Autodesk Inventor part; units mm, degrees
ref_plane "YZ Plane" through (0, 0, 0) normal (1, 0, 0) x (0, 1, 0)
ref_plane "XZ Plane" through (0, 0, 0) normal (0, 1, 0) x (-1, 0, 0)
ref_plane "XY Plane" through (0, 0, 0) normal (0, 0, 1) x (1, 0, 0)
sketch "Sketch1" plane through (0, 0, 0) normal (0, 0, 1) x (1, 0, 0)
  line L0 (0, 0) -> (3, 0)
  line L1 (3, 0) -> (3, 25)
  line L2 (3, 25) -> (0, 25)
  line L3 (0, 25) -> (0, 0)
  line L4 (34, 25) -> (39, 25)
  line L5 (39, 25) -> (39, 0)
  line L6 (39, 0) -> (34, 0)
  line L7 (34, 0) -> (34, 25)
  line L8 (0, 25) -> (39, 25)
  line L9 (39, 25) -> (39, 42)
  line L10 (39, 42) -> (0, 42)
  line L11 (0, 42) -> (0, 25)
  line L12 (34, 25) -> (36, 25)
  line L13 (36, 25) -> (36, 10)
  line L14 (36, 10) -> (34, 10)
  line L15 (34, 10) -> (34, 25)
  point P0 (3, 25)
  point P1 (34, 25)
  dimension "d0" = 3
  dimension "d1" = 25
  dimension "d2" = 5
  dimension "d3" = 25
  dimension "d4" = 31
  dimension "d5" = 39
  dimension "d6" = 17
  dimension "d70" = 2
  dimension "d71" = 15
extrude "Extrusion1" add sketch "Sketch1" along normal blind 17 contours L3 L2 L1 L0 | L11 L10 L9 L4 L8 L2 | L4 L5 L6 L7 L14 L13
sketch "Sketch2" plane through (39, 0, 0) normal (1, 0, 0) x (0, 0, -1)
  line L0 (-17, 28) -> (-17, 42)
  line L1 (0, 42) -> (-17, 42)
  line L2 (-17, 42) -> (0, 42)
  line L3 (0, 42) -> (-17, 28)
  point P0 (0, 0)
  dimension "d9" = 14
extrude "Extrusion2" cut sketch "Sketch2" against normal up to surface (39 mm away)
sketch "Sketch4" plane through (0, 0, 17) normal (0, 0, 1) x (1, 0, 0)
  line L0 (39, 0) -> (39, 42)
  line L1 (20, 42) -> (0, 42)
  line L2 (0, 42) -> (0, 25)
  line L3 (0, 25) -> (20, 25)
  line L4 (20, 25) -> (20, 42)
  circle A0 centre (15, 33.5) radius 3.5
  circle A1 centre (5, 33.5) radius 3.5
  line L5 (3, 25) -> (34, 25)
  line L6 (3, 25) -> (1, 25)
  point P0 (0, 0)
  dimension "d17" = 17
  dimension "d18" = 7
  dimension "d19" = 7
  dimension "d20" = 8.5
  dimension "d22" = 8.5
  dimension "d23" = 5
  dimension "d48" = 5
  dimension "d49" = 20
extrude "Extrusion4" cut sketch "Sketch4" against normal blind 14 contours A0 | A1
sketch "Sketch5" plane through (0, 0, 3) normal (0, 0, 1) x (1, 0, 0)
  arc A0 (15, 37) -> (15, 37) centre (15, 33.5) ccw
  circle A1 centre (15, 33.5) radius 1.5
  circle A2 centre (5, 33.5) radius 3.5
  circle A3 centre (5, 33.5) radius 1.5
  point P0 (0, 0)
  point P1 (32.4191, 39.5294)
  point P2 (27.5809, 39.5294)
  point P3 (22.4191, 39.5294)
  point P4 (17.5809, 39.5294)
  dimension "d26" = 3
  dimension "d27" = 3
extrude "Extrusion5" cut sketch "Sketch5" against normal up to surface (3 mm away) contours A1 | A3
sketch "Sketch10" plane through (0, 0, 17) normal (0, 0, 1) x (1, 0, 0)
  line L0 (39, 42) -> (0, 42)
  line L1 (39, 42) -> (21, 42)
  line L2 (21, 42) -> (21, 35)
  line L3 (39, 28) -> (0, 28)
  line L4 (21, 35) -> (39, 28)
  line L5 (39, 42) -> (39, 28)
  line L6 (39, 28) -> (39, 42)
  point P0 (0, 0)
  dimension "d50" = 18
  dimension "d51" = 7
extrude "Extrusion10" cut sketch "Sketch10" against normal up to surface (17 mm away)
sketch "Sketch11" plane through (39, 0, 17) normal (1, 0, 0) x (0, 0, -1)
  circle A0 centre (8.5, 5) radius 3.75
  line L0 (17, 0) -> (0, 0)
  line L1 (17, 0) -> (17, 28)
  dimension "d54" = 7.5
  dimension "d55" = 5
  dimension "d56" = 8.5
extrude "Extrusion11" cut sketch "Sketch11" against normal up to surface (5 mm away)
sketch "Sketch12" plane through (0, 0, 0) normal (-1, 0, 0) x (0, 0, 1)
  circle A0 centre (8.5, 5) radius 2.5
  line L0 (0, 0) -> (17, 0)
  line L1 (17, 28) -> (17, 0)
  dimension "d59" = 5
  dimension "d60" = 5
  dimension "d61" = 8.5
extrude "Extrusion12" cut sketch "Sketch12" against normal up to surface (3 mm away)
fillet "Fillet2" radius 8.5 4 edges at (1.5, 0, 17) (1.5, 0, 0) (36.5, 0, 17) (36.5, 0, 0)
sketch "Sketch13" plane through (39, 28, 17) normal (1, 0, 0) x (0, 0, -1)
  circle A0 centre (8.5, -23) radius 3.75
  circle A1 centre (8.5, -23) radius 3.5
  circle A2 centre (8.5, -8) radius 2
  circle A3 centre (8.5, -23) radius 3.75
  line L0 (10.4863, -7.7667) -> (12.2244, -22.5625)
  line L1 (6.5137, -7.7667) -> (4.7756, -22.5625)
  point P0 (17, -28)
  dimension "d65" = 4
  dimension "d66" = 15
  dimension "d67" = 0
extrude "Extrusion13" cut sketch "Sketch13" against normal blind 3 contours A0 | A0 L1 A2 L0 | A2 | A1
properties part number "juncao8"
Input: part model. Units: mm. Frame: model coordinates. A direction names the side the tool comes from. Round coordinates to 2 decimals unless told otherwise and drop trailing zeros. Write each loop counter-clockwise with the first axis right and the second up, starting at its lowest first coordinate (ties: lowest second). Pieces come first, ordered by that corner, then holes. Notation, with made-up numbers: (41, 9) - (85, 9) arc R16 ccw to (85, 25) - close; hole circle Ø7 at (47, 48). An arc over 180 degrees is marked (long way). Write item = value, one per line.
(1) Material intervals for probe 1 along Y at (x, z) = (0.9, 8.5); probe 2 along X at (y, z) = (8, 11.25); probe 3 along X at (y, z) = (3, 13.25), sorted ascending.
Geometry check:
probe_1 = 0 to 2.5, 7.5 to 35
probe_2 = 0 to 3, 34 to 36
probe_3 = 0 to 3, 34 to 39
(2) Section query C-C on x = 15. Output: boundary loops of the cut face in (y, z).
Geometry check:
outline = (25, 0) - (32, 0) - (32, 3) - (30, 3) - (30, 14.57) - (28, 17) - (25, 17) - close; (35, 0) - (42, 0) - (37, 6.07) - (37, 3) - (35, 3) - close
(3) Access query for faces 1 (the flat face through (36, 21, 6)), 2 (the flat face through (11.11, 35.1, 8.38)), 3 (the flat face through (37.521, 12.939, 11.343)), 4 (the cylindrical face through (4.241, 30.083, 7.587)), 5 (the flat face through (34, 8, 6)). Directions: +Z, -Z, +X, -X, +Y, -Y. A direction counts if a zero-diameter tool reaches every point of the face in a straight line with its end or side. Return the directions, or none.
Geometry check:
face_1 = +Z, -Z
face_2 = +Z, +X, -X, +Y
face_3 = +X
face_4 = +Z
face_5 = +Z, -Z, -Y
(4) Section query D-D on z = 1. Output: boundary loops of the cut face in (x, y), then the cut area to 3 significant figures.
Geometry check:
outline = (0, 4.5) - (3, 4.5) - (3, 25) - (36, 25) - (36, 10) - (34, 10) - (34, 4.5) - (39, 4.5) - (39, 28) - (21, 35) - (21, 41.18) - (0, 41.18) - close; hole circle Ø3 at (5, 33.5); hole circle Ø3 at (15, 33.5)
area = 577 mm^2
(5) Pull-direction query (X, two-part tool) for faces 6 (the flat face through (39, 17, 12)), 7 (the cylindrical face through (14.241, 30.083, 7.587)), 8 (the cylindrical face through (1.52, 2.56, 14.58)); classes: +X half, -X half, draft (parallel to the pull), parting line (faces both ways), or undercut.
Geometry check:
face_6 = +X half
face_7 = undercut
face_8 = draft
(6) Contact query for flat-ended pins moving along their axis: pin 1 Ø8 at (x, z) = (15.5, 15) entering from -Y; pin 2 Ø2 at (x, z) = (35, 12.5) entering from +Y; pin 3 Ø10 at (x, y) = (30, 34) entering from +Z. Output: stop coordinate, or through.
Geometry check:
pin_1 = 25
pin_2 = 29.94
pin_3 = 15.79
(7) Section query A-A on y = 34. Output: boundary loops of the cut face in (x, z), then the cut area to 3 significant figures.
Geometry check:
outline = (0, 0) - (3.59, 0) - (3.59, 3) - (1.54, 3) - (1.54, 9.71) - (0, 9.71) - close; (6.41, 0) - (13.59, 0) - (13.59, 3) - (11.54, 3) - (11.54, 9.71) - (8.46, 9.71) - (8.46, 3) - (6.41, 3) - close; (16.41, 0) - (23.57, 0) - (23.57, 9.71) - (18.46, 9.71) - (18.46, 3) - (16.41, 3) - close
area = 119 mm^2
(8) Section query B-B on z = 8. Output: boundary loops of the cut face in (x, y).
Geometry check:
outline = (0, 0.01) - (3, 0.01) - (3, 2.55) - (0, 2.55) - close; (0, 7.45) - (3, 7.45) - (3, 25) - (36, 25) - (36, 21.94) - (39, 21.94) - (39, 28) - (21, 35) - (21, 35.41) - (17.93, 35.41) arc R3.5 cw (long way) to (12.07, 35.41) - (7.93, 35.41) arc R3.5 cw (long way) to (2.07, 35.41) - (0, 35.41) - close; (34, 0.01) - (39, 0.01) - (39, 1.28) - (34, 1.28) - close; (34, 8.72) - (36, 8.72) - (36, 10) - (34, 10) - close
